```python
from build123d import *

# Parameters (mm, degrees)
BOSS_EXTRUDE1_DEPTH = 3
SKETCH2_R           = 10
CUT_EXTRUDE1_DEPTH  = 7


with BuildPart() as part:
    # Sketch1 → Boss-Extrude1 (new body, symmetric)
    with BuildSketch(Plane(origin=(0, 0, 0), x_dir=(0, 0, -1), z_dir=(1, 0, 0))):
        with BuildLine():
            ThreePointArc((-12.5, -170.38750305), (0, -224.5), (12.5, -170.38750305))
            Line((12.5, -170.38750305), (12.5, 170.38750305))
            ThreePointArc((12.5, 170.38750305), (13.38309417, 170.837671204), (14.25, 171.318275992))
            Line((14.25, 171.318275992), (12.5, 174.349364905))
            Line((12.5, 174.349364905), (12.5, 174.928692494))
            ThreePointArc((12.5, 174.928692494), (0, 220.5), (-12.5, 174.928692494))
            Line((-12.5, 174.928692494), (-12.5, 174.349364905))
            Line((-12.5, 174.349364905), (-14.25, 171.318275992))
            ThreePointArc((-14.25, 171.318275992), (-13.38309417, 170.837671204), (-12.5, 170.38750305))
            Line((-12.5, 170.38750305), (-12.5, -170.38750305))
        make_face()
    extrude(amount=BOSS_EXTRUDE1_DEPTH, both=True)

    # Sketch2 → Cut-Extrude1 (cut, through all)
    with BuildSketch(Plane(origin=(3, 0, 0), x_dir=(0, 0, -1), z_dir=(1, 0, 0))):
        with Locations((0, -196)):
            Circle(SKETCH2_R)
        with Locations((0, 196)):
            Circle(SKETCH2_R)
    extrude(amount=-CUT_EXTRUDE1_DEPTH, mode=Mode.SUBTRACT)


solid = part.part
```
The listing builds one solid part. Answer for the finished solid, in the listing's coordinates (mm). Give positions to 0.01 mm unless a question says otherwise; leave off trailing zeros. Order: outer loops, then holes, each group sorted by start corner. A loop starts at its lowest first (then second) coordinate and runs counter-clockwise, first axis right, second up.
1) Determine the mould class of faces 1 (the face through (-3, 1, 0)), 2 (the face through (0.04, -205.76, 2.17)) for opening direction Y: pulls with the +Y half, pulls with the -Y half, needs draft (parallel to the pull), parting line crosses it, or undercut.
Reported:
face 1: needs draft
face 2: undercut
2) Given P1, Ø1.5, axis at x = -1.5, y = 158.5, coming from the +Z side; P2, Ø3, axis at x = 0, z = 6.5, coming from the -Y side; P3, Ø0.6, axis at x = 1.5, y = 174.5, coming from the +Z side, each flat-ended and moving along its own axis, determine where each tip first touches the part or whether it passes through.
Reported:
P1: stops at z = 12.5
P2: stops at y = -224.06
P3: stops at z = 12.59
3) Find section D-D on z = 18. Write down the section's boundary in (x, y), then the cut area to 3 significant figures.
Reported:
outline: (-3, -218.1) - (3, -218.1) - (3, -173.9) - (-3, -173.9) - close; (-3, 179.38) - (3, 179.38) - (3, 212.62) - (-3, 212.62) - close
area: 465 mm2
4) Consider line 1 along Y through (x, z) = (0.4, 0); line 2 along Y through (x, z) = (1.35, -2); line 3 along Z through (x, y) = (2.2, -130.5). Determine where each line is inside the solid, lowest interval first.
Reported:
line 1: y = -224.5 to -206, -186 to 186, 206 to 220.5
line 2: y = -224.43 to -205.8, -186.2 to 186.2, 205.8 to 220.42
line 3: z = -12.5 to 12.5
5) Find section A-A on z = 0. Write down the section's boundary in (x, y).
Reported:
outline: (-3, -224.5) - (3, -224.5) - (3, -206) - (-3, -206) - close; (-3, -186) - (3, -186) - (3, 186) - (-3, 186) - close; (-3, 206) - (3, 206) - (3, 220.5) - (-3, 220.5) - close
6) Find section B-B on y = -196. Write down the section's boundary in (x, z), then the cut area to 3 significant figures.
Reported:
outline: (-3, -28.5) - (3, -28.5) - (3, -10) - (-3, -10) - close; (-3, 10) - (3, 10) - (3, 28.5) - (-3, 28.5) - close
area: 222 mm2
7) Find section C-C on x = -1.95. Write down the section's boundary in (y, z).
Reported:
outline: (-170.39, -12.5) - (170.39, -12.5) arc R28.5 ccw to (171.32, -14.25) - (174.35, -12.5) - (174.93, -12.5) arc R24.5 ccw (long way) to (174.93, 12.5) - (174.35, 12.5) - (171.32, 14.25) arc R28.5 ccw to (170.39, 12.5) - (-170.39, 12.5) arc R28.5 ccw (long way) to start; hole circle Ø20 at (-196, 0); hole circle Ø20 at (196, 0)
